```python
from build123d import *

# Parameters (mm, degrees)
F1_DEPTH = 4.25
F2_R     = 2


with BuildPart() as f1:
    # F0 (on Top) → F1 (new body, symmetric)
    with BuildSketch(Plane.XY):
        Polygon((-26.5, -42.5), (26.5, -42.5), (26.5, 42.5), (3, 42.5), (3, 41.5), (-3, 41.5), (-3, 42.5), (-26.5, 42.5), align=None)
    extrude(amount=F1_DEPTH, both=True)

    # F2
    f2_edges = [f1.edges().sort_by_distance(p)[0] for p in [
        (-26.5, -42.5, 0),
        (26.5, -42.5, 0),
        (26.5, 42.5, 0),
        (-26.5, 42.5, 0),
    ]]
    fillet(f2_edges, radius=F2_R)


solid = f1.part
```
CAD build for the part. Positions are in the model's coordinates, mm. Give positions to 0.01 mm unless a question says otherwise; leave off trailing zeros. Put each result on its own line as item: value. Start each with the question number.
(1) Mould opens along X. For faces 1 (the flat face through (0, 1, 4.25)), 2 (the cylindrical face through (-25.93, 41.9, -0.06)), 3 (the flat face through (0, 41.5, 0)) say: +X half, -X half, draft (parallel to the pull), parting line (faces both ways), or undercut.
(2) Flat gauge pins, fed straight in: pin 1 Ø0.8 at (y, z) = (42, -2) entering from +X; pin 2 Ø0.5 at (y, z) = (42, -2) entering from -X; pin 3 Ø1.8 at (x, z) = (-0.5, 1.5) entering from +Y. Where does each tip first touch, or does it go through?
(3) Drill centre line: line 1 along Y through (x, z) = (-1.5, 2). Where is it in solid material? Low to high.
Check result:
1. face 1: draft
1. face 2: -X half
1. face 3: undercut
2. pin 1: stops at x = 26.17
2. pin 2: stops at x = -26.06
2. pin 3: stops at y = 41.5
3. line 1: y = -42.5 to 41.5
